Verification items for the finished model (mm, model axes). Coordinates: 2 decimals unless noted, no trailing zeros. Order: outer loops, then holes, each group sorted by start corner. A loop starts at its lowest first (then second) coordinate and runs counter-clockwise, first axis right, second up. Notation, with made-up numbers: M -2,-2 L 12,-2 A18 cw 12,25 Z; hole C 60,50 d9. An arc over 180 degrees is marked long. Write item = value, one per line.
Autodesk Inventor part; units mm, degrees
ref_plane "Arbeitsebene1" through (0, 0, 300) normal (0, 0, 1) x (1, 0, 0)
ref_plane "YZ Plane" through (0, 0, 0) normal (1, 0, 0) x (0, 1, 0)
ref_plane "XZ Plane" through (0, 0, 0) normal (0, 1, 0) x (-1, 0, 0)
sketch "Skizze1" plane through (0, 0, 0) normal (0, 0, 1) x (1, 0, 0)
  line L0 (0, 0) -> (10, 0)
  line L1 (10, 0) -> (10, 10)
  line L2 (10, 10) -> (0, 10)
  line L3 (0, 10) -> (0, 0)
extrude "Extrusion1" add sketch "Skizze1" along normal blind 300
sketch "Skizze2" plane through (0, 0, 0) normal (0, 0, 1) x (1, 0, 0)
  line L0 (0, 0) -> (4, 0)
  line L1 (4, 0) -> (4, 4)
  line L2 (4, 4) -> (0, 4)
  line L3 (0, 4) -> (0, 0)
extrude "Extrusion2" cut sketch "Skizze2" along normal blind 300
sketch "Skizze3" plane through (0, 0, 0) normal (0, 0, 1) x (1, 0, 0)
  line L0 (-3, 6) -> (3, 6)
  line L1 (3, 6) -> (3, 10)
  line L2 (3, 10) -> (-3, 10)
  line L3 (-3, 10) -> (-3, 6)
extrude "Extrusion3" cut sketch "Skizze3" along normal blind 300
sketch "Skizze4" plane through (0, 0, 0) normal (0, 0, 1) x (1, 0, 0)
  line L0 (-3, -10) -> (3, -10)
  line L1 (3, -10) -> (3, -6)
  line L2 (3, -6) -> (-3, -6)
  line L3 (-3, -6) -> (-3, -10)
extrude "Extrusion4" cut sketch "Skizze4" along normal blind 300
sketch "Skizze5" plane through (0, 0, 0) normal (0, 0, 1) x (1, 0, 0)
  line L0 (-10, -3) -> (-6, -3)
  line L1 (-6, -3) -> (-6, 3)
  line L2 (-6, 3) -> (-10, 3)
  line L3 (-10, 3) -> (-10, -3)
extrude "Extrusion5" cut sketch "Skizze5" along normal blind 300
sketch "Skizze6" plane through (0, 0, 0) normal (0, 0, 1) x (1, 0, 0)
  line L0 (6, -3) -> (10, -3)
  line L1 (10, -3) -> (10, 3)
  line L2 (10, 3) -> (6, 3)
  line L3 (6, 3) -> (6, -3)
extrude "Extrusion6" cut sketch "Skizze6" along normal blind 300
ref_plane "Arbeitsebene1" through (0, 0, 300) normal (0, 0, 1) x (1, 0, 0)
sketch "Skizze7" plane through (0, 0, 0) normal (0, 0, 1) x (1, 0, 0)
  circle A0 centre (0, 0) radius 2.5
extrude "Extrusion7" cut sketch "Skizze7" along normal blind 10
sketch "Skizze8" plane through (0, 0, 300) normal (0, 0, 1) x (1, 0, 0)
  circle A0 centre (0, 0) radius 2.5
extrude "Extrusion8" cut sketch "Skizze8" along normal blind 10
properties part number "Aluprofil_20x20_L300"
Item 1: Scan lines: L1, parallel to Y at x = 6.25, z = 130.5; L2, parallel to Y at x = 2, z = 126.5. Record each from-to range of solid material in increasing order. Write a range as from..to.
Report:
L1 = 3..10
L2 = 4..6
Item 2: Sectioned sample at B-B, the plane y = 1.5. Enter the section's corners in (x, z).
Report:
outline = M 4,0 L 6,0 L 6,300 L 4,300 Z
Item 3: Sectioned sample at A-A, the plane z = 129. Enter the section's corners in (x, y), then the cut area to 3 significant figures.
Report:
outline = M 0,4 L 4,4 L 4,0 L 6,0 L 6,3 L 10,3 L 10,10 L 3,10 L 3,6 L 0,6 Z
area = 60.0 mm^2
Item 4: Sectioned sample at C-C, the plane x = 8.5. Enter the section's corners in (y, z).
Report:
outline = M 3,0 L 10,0 L 10,300 L 3,300 Z
Item 5: Gauge pin test, flat ends, axial feed: pin 1 (3 mm diameter, centred on y = 8, z = 187, fed in from -X); pin 2 (2 mm diameter, centred on y = 2.5, z = 104, fed in from -X); pin 3 (0.9 mm diameter, centred on x = 1, z = 215, fed in from +Y). Record the tip position at first contact, or that the pin passes through.
Report:
pin_1 = 3
pin_2 = 4
pin_3 = 6
